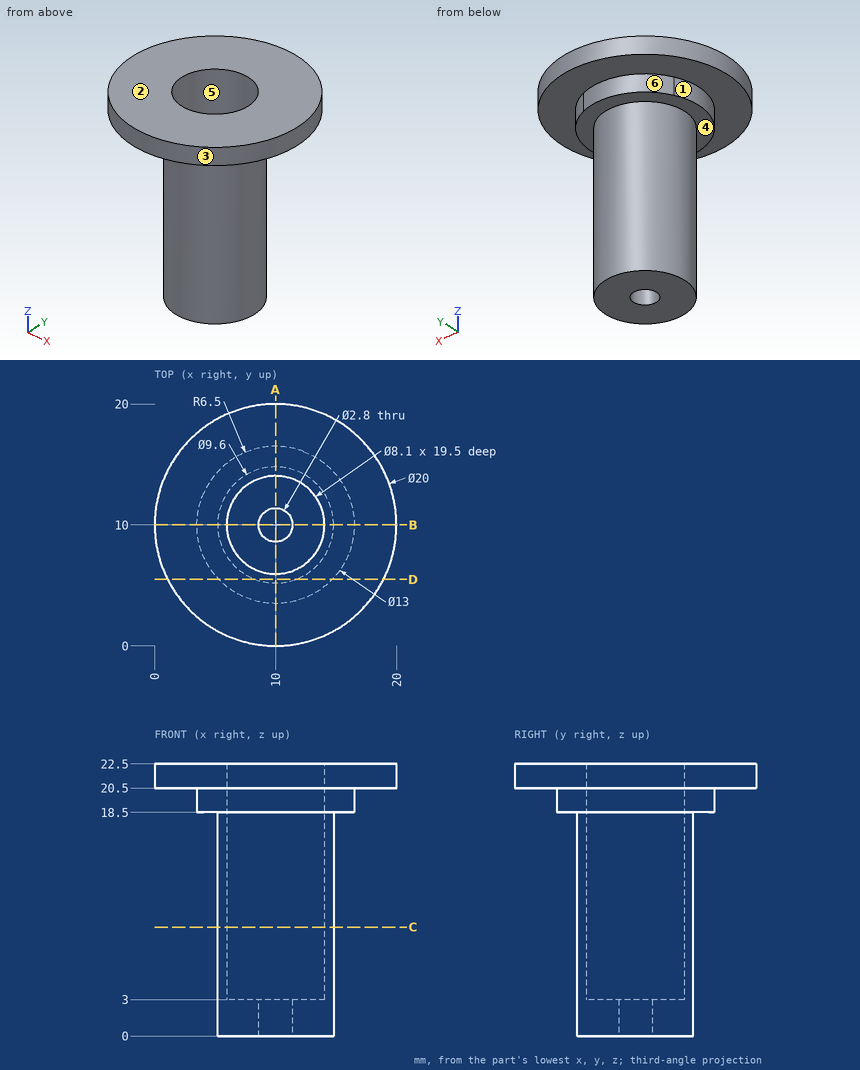
Part print with two shaded views. Sizes in mm from the minimum x, y, z corner. A direction names the side the tool comes from. Coordinates: 2 decimals unless noted, no trailing zeros. Order: outer loops, then holes, each group sorted by start corner. A loop starts at its lowest first (then second) coordinate and runs counter-clockwise, first axis right, second up. Notation, with made-up numbers: (-21, -38) - (8, -38) arc R32 cw to (8, -8) - close; hole circle Ø10 at (38.25, 53). An arc over 180 degrees is marked (long way). Write item = value, one per line. Start each with the question number.
1) Wall check: line 1 along Y through (x, z) = (10, 1.8); line 2 along Y through (x, z) = (9.75, 3.75); line 3 along Z through (x, y) = (19, 7). Give the ranges that are in metal, low to high. Write a range as from..to.
2) Saw through at D-D on y = 5.5. Write the cut outline in (x, z).
3) Two-plate mould, pull along Y, no slides. Class the marked faces 3, 4, 5 and 6: pulls with the +Y half, pulls with the -Y half, needs draft (parallel to the pull), parting line crosses it, or undercut.
4) 3-axis set-ups, long thin cutter, end or side, ignore diameter. For the marked faces 1 and 2: which of +Z, -Z, +X, -X, +Y, -Y reach the whole face in a straight line?
5) Saw through at C-C on z = 9. Write the cut outline in (x, y).
6) Saw through at A-A on x = 10. Write the cut outline in (y, z).
7) Flat gauge pins, fed straight in: pin 1 Ø4 at (x, y) = (9, 10) entering from +Z; pin 2 Ø4 at (x, z) = (8, 9) entering from -Y; pin 3 Ø2 at (y, z) = (11.5, 6.5) entering from -X. Where does each tip first touch, or does it go through?
From the geometry:
q1.line_1 = 5.2..8.6, 11.4..14.8
q1.line_2 = 5.21..5.96, 14.04..14.79
q1.line_3 = 20.5..22.5
q2.outline = (1.07, 20.5) - (5.31, 20.5) - (5.31, 18.5) - (8.33, 18.5) - (8.33, 0) - (11.67, 0) - (11.67, 18.5) - (14.69, 18.5) - (14.69, 20.5) - (18.93, 20.5) - (18.93, 22.5) - (1.07, 22.5) - close
q3.face_3 = parting line crosses it
q3.face_4 = needs draft
q3.face_5 = undercut
q3.face_6 = pulls with the +Y half
q4.face_1 = -Z
q4.face_2 = +Z, +X, -X, +Y, -Y
q5.outline = circle Ø9.6 at (10, 10); hole circle Ø8.1 at (10, 10)
q6.outline = (0, 20.5) - (3.5, 20.5) - (3.5, 18.5) - (5.2, 18.5) - (5.2, 0) - (8.6, 0) - (8.6, 3) - (5.95, 3) - (5.95, 22.5) - (0, 22.5) - close; (11.4, 0) - (14.8, 0) - (14.8, 18.5) - (16.5, 18.5) - (16.5, 20.5) - (20, 20.5) - (20, 22.5) - (14.05, 22.5) - (14.05, 3) - (11.4, 3) - close
q7.pin_1 = 3
q7.pin_2 = 5.2
q7.pin_3 = 5.23
